from build123d import *

# Parameters (mm, degrees)
F0_W     = 21.082
F0_H     = 88.9
F0_W_2   = 21.336
F1_DEPTH = 20.32
F2_DEPTH = 10.16
F3_R     = 2.54
F5_DEPTH = 88.9


# Not quite as in the source:
# - the program builds the solid bodies; features that only make, move or delete a surface that nothing else refers to are left out


with BuildPart() as f1:
    # F0 (on Top) → F1 (new body)
    with BuildSketch(Plane.XY):
        with Locations((-23.6977891486, 3.6070292577)):
            Rectangle(F0_W, F0_H)
        with Locations((-2.6157891486, 3.6070292577)):
            Rectangle(F0_W, F0_H)
        with Locations((18.5932108514, 3.6070292577)):
            Rectangle(F0_W_2, F0_H)
    extrude(amount=F1_DEPTH)

    # F0 (on Top) → F2 (cut)
    with BuildSketch(Plane.XY):
        with Locations((-2.6157891486, 3.6070292577)):
            Rectangle(F0_W, F0_H)
    extrude(amount=F2_DEPTH, mode=Mode.SUBTRACT)

    # F3 (on face) → F5 (cut)
    with BuildSketch(Plane(origin=(0, 48.0570292577, 0), x_dir=(-1, 0, 0), z_dir=(0, 1, 0))):
        with Locations((2.6157891486, 14.9523410946)):
            Circle(F3_R)
    extrude(amount=-F5_DEPTH, mode=Mode.SUBTRACT)


solid = f1.part
For this review, take the finished solid that the model builds, in its own axes (mm). A direction names the side the tool comes from. Coordinates: 2 decimals unless noted, no trailing zeros. Order: outer loops, then holes, each group sorted by start corner. A loop starts at its lowest first (then second) coordinate and runs counter-clockwise, first axis right, second up. Notation, with made-up numbers: (6, 82) - (49, 82) arc R30 ccw to (49, 116) - close; hole circle Ø1 at (-13.5, 61.25). An arc over 180 degrees is marked (long way). Use one line per item in the form item = value.
Q1. Draft analysis for pull direction X (two halves, no side actions). For faces 1 (the flat face through (29.261, 3, 10)), 2 (the flat face through (-34.239, 3, 10)), 3 (the flat face through (-3, 4, 10.16)), state which applies: +X half, -X half, draft (parallel to the pull), parting line (faces both ways), or undercut.
Checked values:
face_1 = +X half
face_2 = -X half
face_3 = undercut
Q2. Consider section A-A (z = 6.5). Give the boundary of the cut face in (x, y).
Checked values:
outline = (-34.24, -40.84) - (-13.16, -40.84) - (-13.16, 48.06) - (-34.24, 48.06) - close; (7.93, -40.84) - (29.26, -40.84) - (29.26, 48.06) - (7.93, 48.06) - close
Q3. For faces 4 (the flat face through (-13.157, 3, 5)), 5 (the flat face through (-24, 4, 0)), list the 3-axis set-ups (+Z, -Z, +X, -X, +Y, -Y) from which the entire face can be reached by the end or side of a thin tool; tool diameter is ignored.
Checked values:
face_4 = -Z, +Y, -Y
face_5 = -Z, +X, -X, +Y, -Y
Q4. Consider section D-D (x = 6.5). Give the boundary of the cut face in (y, z), then the cut area to 3 significant figures.
Checked values:
outline = (-40.84, 10.16) - (48.06, 10.16) - (48.06, 20.32) - (-40.84, 20.32) - close
area = 903 mm2
Q5. Consider section C-C (y = -21). Give the boundary of the cut face in (x, z), then the cut area to 3 significant figures.
Checked values:
outline = (-34.24, 0) - (-13.16, 0) - (-13.16, 10.16) - (7.93, 10.16) - (7.93, 0) - (29.26, 0) - (29.26, 20.32) - (-34.24, 20.32) - close; hole circle Ø5.08 at (-2.62, 14.95)
area = 1,060 mm2
Q6. For probe 1 along X at (y, z) = (32, 3.5); probe 2 along Z at (x, y) = (-2.5, -14); probe 3 along X at (y, z) = (-28, 15.5), list the stretches that pass through material, from the lowest coordinate up. Write a range as from..to.
Checked values:
probe_1 = -34.24..-13.16, 7.93..29.26
probe_2 = 10.16..12.41, 17.49..20.32
probe_3 = -34.24..-5.1, -0.14..29.26
Q7. Consider section B-B (x = -2). Give the boundary of the cut face in (y, z), then the cut area to 3 significant figures.
Checked values:
outline = (-40.84, 10.16) - (48.06, 10.16) - (48.06, 12.49) - (-40.84, 12.49) - close; (-40.84, 17.42) - (48.06, 17.42) - (48.06, 20.32) - (-40.84, 20.32) - close
area = 465 mm2
Q8. For P1, Ø12, axis at x = -7.5, y = 26, coming from the -Z side; P2, Ø6.5, axis at x = -1.5, y = -13, coming from the -Z side, all flat-tipped, find the tip position at first contact; note any pin that passes through.
Checked values:
P1 = 0
P2 = 10.16
